Can you work these out from the model? Positions are in its coordinate system, mm. A direction names the side the tool comes from. Round coordinates to 2 decimals unless told otherwise and drop trailing zeros. Write each loop counter-clockwise with the first axis right and the second up, starting at its lowest first coordinate (ties: lowest second). Pieces come first, ordered by that corner, then holes.
Q1. For faces 4 (the flat face through (10, -80, 6)), 5 (the flat face through (15, -81, 1.5)), 6 (the flat face through (0, -43, 1)), which set-ups out of +Z, -Z, +X, -X, +Y, -Y let a thin tool reach every point of the face, with its end or its side?
Q2. If we section it at B-B (z = 6.5): Please give me the cut outline in (x, y).
Q3. We'd pull the mould along X, two halves only. Please class faces 1 (the cylindrical face through (4.93, -80.76, 4.95)), 2 (the flat face through (10, -81.5, 6)), 3 (the cylindrical face through (8.859, -1.203, 0.76)): +X half, -X half, draft (parallel to the pull), parting line (faces both ways), or undercut.
Q4. If we section it at D-D (x = 1.5): Please give me the cut outline in (y, z).
Q5. Please list where these lines run through material, in increasing order: line 1 along X through (y, z) = (-80.25, 6.5); line 2 along Z through (x, y) = (15, -80.8); line 3 along Z through (x, y) = (5, -80.9).
Q6. If we section it at C-C (y = -37): Please give me the cut outline in (x, z), plus the area to 3 significant figures.
Q7. If we section it at A-A (x = 15): Please give me the cut outline in (y, z), plus the area to 4 significant figures.
Q8. I'm going to push flat-ended pins straight in: pin 1 Ø3 at (x, z) = (5.5, 4.5) entering from +Y; pin 2 Ø0.8 at (x, y) = (15.5, -80.5) entering from -Z; pin 3 Ø1.2 at (y, z) = (-37, 0.5) entering from +X. Where does each tip first touch, or does it pass through?
Autodesk Inventor part; units mm, degrees
ref_plane "YZ Plane" through (0, 0, 0) normal (1, 0, 0) x (0, 1, 0)
ref_plane "XZ Plane" through (0, 0, 0) normal (0, 1, 0) x (-1, 0, 0)
ref_plane "XY Plane" through (0, 0, 0) normal (0, 0, 1) x (1, 0, 0)
sketch "スケッチ1" plane through (0, 0, 0) normal (0, 0, 1) x (1, 0, 0)
  line L0 (0, 0) -> (10, 0)
  line L1 (10, 0) -> (10, -80)
  line L2 (10, -80) -> (0, -80)
  line L3 (0, -80) -> (0, 0)
  dimension "d0" = 10
  dimension "d1" = 80
extrude "押し出し1" add sketch "スケッチ1" along normal blind 1.5
fillet "フィレット1" radius 4 2 edges at (10, 0, 0.75) (0, 0, 0.75)
sketch "スケッチ2" plane through (0, -80, 0) normal (0, -1, 0) x (1, 0, 0)
  line L0 (0, 1.5) -> (10, 1.5)
  line L1 (10, 1.5) -> (10, 0)
  line L2 (10, 0) -> (0, 0)
  line L3 (0, 0) -> (0, 1.5)
extrude "押し出し2" add sketch "スケッチ2" along normal blind 1.5
sketch "スケッチ4" plane through (0, 0, 1.5) normal (0, 0, 1) x (1, 0, 0)
  line L0 (20, -81.5) -> (-10, -81.5)
  line L1 (-10, -81.5) -> (-10, -80)
  line L2 (-10, -80) -> (20, -80)
  line L3 (20, -80) -> (20, -81.5)
  point P0 (0, 0)
  dimension "d10" = 30
  dimension "d11" = 1.5
extrude "押し出し4" add sketch "スケッチ4" along normal blind 10
sketch "スケッチ6" plane through (-10, -80, 1.5) normal (0, 1, 0) x (1, 0, 0)
  line L0 (0, -10) -> (10, -10)
  line L1 (10, -10) -> (10, 0)
  line L2 (10, 0) -> (0, 0)
  line L3 (0, 0) -> (0, -10)
  point P0 (10, 1.5)
extrude "押し出し6" cut sketch "スケッチ6" against normal blind 10
sketch "スケッチ8" plane through (10, -80, 1.5) normal (0, 1, 0) x (1, 0, 0)
  line L0 (10, 0) -> (10, -10)
  line L1 (10, -10) -> (-10, -10)
  point P0 (-10, 1.5)
  point P1 (-5, -5)
  point P2 (5, -5)
  dimension "d25" = 5
  dimension "d26" = 5
  dimension "d27" = 10
hole "穴1" at (5, -80, 6.5) at (15, -80, 6.5) direction (0, -1, 0) diameter 3.1 depth 8 tip angle 118
properties part number "Fork 1 left ver2" material "アルミニウム 5052 H32"
A:
1. face 4: +Z, +X, -X, +Y
1. face 5: -Z, +X, +Y, -Y
1. face 6: +Z, -Z, -X, +Y, -Y
2. outline: (0, -81.5) - (3.45, -81.5) - (3.45, -80) - (0, -80) - close; (6.55, -81.5) - (13.45, -81.5) - (13.45, -80) - (6.55, -80) - close; (16.55, -81.5) - (20, -81.5) - (20, -80) - (16.55, -80) - close
3. face 1: undercut
3. face 2: draft
3. face 3: +X half
4. outline: (-81.5, 0) - (-0.88, 0) - (-0.88, 1.5) - (-80, 1.5) - (-80, 11.5) - (-81.5, 11.5) - close
5. line 1: x = 0 to 3.45, 6.55 to 13.45, 16.55 to 20
5. line 2: z = 1.5 to 4.95, 8.05 to 11.5
5. line 3: z = 0 to 4.95, 8.05 to 11.5
6. outline: (0, 0) - (10, 0) - (10, 1.5) - (0, 1.5) - close
6. area: 15.0 mm2
7. outline: (-81.5, 1.5) - (-80, 1.5) - (-80, 4.95) - (-81.5, 4.95) - close; (-81.5, 8.05) - (-80, 8.05) - (-80, 11.5) - (-81.5, 11.5) - close
7. area: 10.35 mm2
8. pin 1: stops at y = -80
8. pin 2: stops at z = 1.5
8. pin 3: stops at x = 10
